Could you check a few things on this model? Use its own coordinates, in mm. Face numbers are marked on the shaded views. A direction names the side the tool comes from. Give positions to 0.01 mm unless a question says otherwise; leave off trailing zeros. Loops run counter-clockwise (first coordinate to the right, second up) from the corner with the lowest first, then second, coordinate; pieces in that order, holes last. Notation, with made-up numbers: (-25, 68) - (-16, 68) arc R17 cw to (-16, 83) - close; hole circle Ø10 at (-26.5, -30.75). An arc over 180 degrees is marked (long way). Write each question's results on one line, items separated by ' | '. Start each with the question number.
1) I want a section at B-B, the plane y = 9.1. Write out the boundary of the cut face in (x, z), and give its area (3 significant figures).
2) If we mould it in two halves opening along Y, with no side actions, what happens to the marked faces 3, 4 and 5? For each: +Y half, -Y half, draft (parallel to the pull), parting line (faces both ways), or undercut.
3) I want a section at C-C, the plane x = 30.9. Write out the boundary of the cut face in (y, z).
4) If I drill on probe 1 along Y at (x, z) = (30.9, 38.15); probe 2 along Z at (x, y) = (14, 36.5); probe 3 along X at (y, z) = (20.5, 37.5), over which ranges is the centre line in solid material (lowest first)? Write a range as [from, to].
5) On a 3-axis mill with a long thin cutter (end or side, diameter ignored), from which of +Z, -Z, +X, -X, +Y, -Y can I reach the whole of each face in a straight line? I mean the marked faces 1 and 2. Say none if no direction works.
6) I want a section at D-D, the plane y = 19.5. Write out the boundary of the cut face in (x, z).
7) I want a section at A-A, the plane x = 5.1. Write out the boundary of the cut face in (y, z).
8) I'm going to push flat-ended pins straight in: pin 1 (4 mm diameter, centred on x = 5.1, y = 9.1, fed in from +Z); pin 2 (2.5 mm diameter, centred on x = 19.5, z = 40.5, fed in from -Y); pin 3 (6 mm diameter, centred on x = 25, y = 17, fed in from -Z); pin 4 (4.5 mm diameter, centred on x = 6, z = 34, fed in from -Y). Where does each tip first touch, or does it pass through?
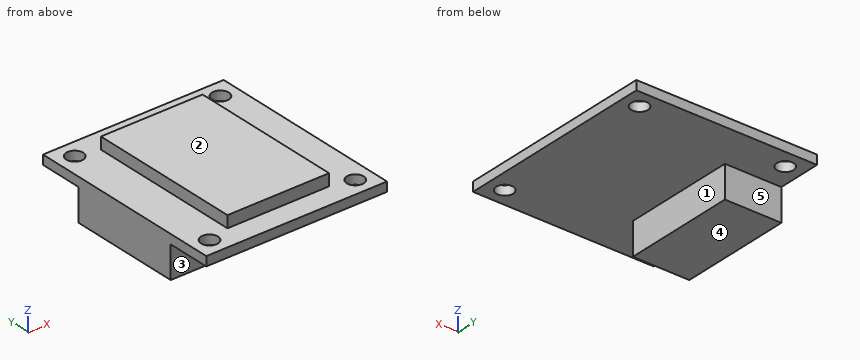
from build123d import *

# Parameters (mm, degrees)
SKETCH042_W  = 32
SKETCH042_H  = 35.5
SKETCH042_R  = 1.5
PAD025_DEPTH = 1.65
SKETCH043_W  = 18
SKETCH043_H  = 27.5
PAD026_DEPTH = 2.1
SKETCH044_W  = 10
SKETCH044_H  = 20
PAD027_DEPTH = 5.7


with BuildPart() as part:
    # Sketch042 → Pad025 (new body)
    with BuildSketch(Plane.XY):
        with Locations((16, 17.75)):
            Rectangle(SKETCH042_W, SKETCH042_H)
        with Locations((3.1, 32.4)):
            Circle(SKETCH042_R, mode=Mode.SUBTRACT)
        with Locations((28.9, 32.4)):
            Circle(SKETCH042_R, mode=Mode.SUBTRACT)
        with Locations((28.9, 3.1)):
            Circle(SKETCH042_R, mode=Mode.SUBTRACT)
        with Locations((3.1, 3.1)):
            Circle(SKETCH042_R, mode=Mode.SUBTRACT)
    extrude(amount=PAD025_DEPTH)

    # Sketch043 (on Face10 of Pad025) → Pad026 (join)
    with BuildSketch(Plane.XY.offset(1.65)):
        with Locations((16, 17.75)):
            Rectangle(SKETCH043_W, SKETCH043_H)
    extrude(amount=PAD026_DEPTH)

    # Sketch044 (on Face4 of Pad026) → Pad027 (join)
    with BuildSketch(Plane(origin=(0, 0, 0), x_dir=(1, 0, 0), z_dir=(0, 0, -1))):
        with Locations((5, -17.75)):
            Rectangle(SKETCH044_W, SKETCH044_H)
    extrude(amount=PAD027_DEPTH)


with BuildPart() as part_1:
    # Body006 placement: moved
    add(part.part.moved(Location((2, 6, 37.75))))


solid = part_1.part
Answers:
1) outline: (2, 37.75) - (3.6, 37.75) - (3.6, 39.4) - (2, 39.4) - close; (6.6, 37.75) - (29.4, 37.75) - (29.4, 39.4) - (6.6, 39.4) - close; (32.4, 37.75) - (34, 37.75) - (34, 39.4) - (32.4, 39.4) - close | area: 42.9 mm2
2) face 3: -Y half | face 4: draft | face 5: +Y half
3) outline: (6, 37.75) - (7.6, 37.75) - (7.6, 39.4) - (6, 39.4) - close; (10.6, 37.75) - (36.9, 37.75) - (36.9, 39.4) - (10.6, 39.4) - close; (39.9, 37.75) - (41.5, 37.75) - (41.5, 39.4) - (39.9, 39.4) - close
4) probe 1: y = [6, 7.6], [10.6, 36.9], [39.9, 41.5] | probe 2: z = [37.75, 41.5] | probe 3: x = [2, 12]
5) face 1: -Z, +X, +Y, -Y | face 2: +Z, +X, -X, +Y, -Y
6) outline: (2, 32.05) - (12, 32.05) - (12, 37.75) - (34, 37.75) - (34, 39.4) - (27, 39.4) - (27, 41.5) - (9, 41.5) - (9, 39.4) - (2, 39.4) - close
7) outline: (6, 37.75) - (7.6, 37.75) - (7.6, 39.4) - (6, 39.4) - close; (10.6, 37.75) - (13.75, 37.75) - (13.75, 32.05) - (33.75, 32.05) - (33.75, 37.75) - (36.9, 37.75) - (36.9, 39.4) - (10.6, 39.4) - close; (39.9, 37.75) - (41.5, 37.75) - (41.5, 39.4) - (39.9, 39.4) - close
8) pin 1: stops at z = 39.4 | pin 2: stops at y = 6 | pin 3: stops at z = 37.75 | pin 4: stops at y = 13.75
